Part model, mm, in its own coordinate system. Face numbers are marked on the shaded views. A direction names the side the tool comes from. Give positions to 0.01 mm unless a question says otherwise; leave off trailing zeros. Write each loop counter-clockwise with the first axis right and the second up, starting at its lowest first coordinate (ties: lowest second). Pieces come first, ordered by that corner, then holes. Notation, with made-up numbers: M -35,42 L 19,42 A33 cw 19,76 Z; hole C -7.75,-10 d3. An arc over 180 degrees is marked long. Use CSV: the item, a comma, the result in double quotes. Start each with the question number.
Item 1: Cut at A-A (x = -23). List the corners of the cut face in (y, z).
Item 2: Drill centre lines: line 1 (Z direction, x = -1, y = 37.5); line 2 (X direction, y = 141, z = 12); line 3 (Y direction, x = -45.5, z = 38). Where is each one in solid material? Low to high. Write a range as [from, to].
Item 3: Which spindle directions (+Z, -Z, +X, -X, +Y, -Y) get a long thin tool onto all of the face, cutting with end or side? Do the marked faces 1, 2, 3 and 4. Say none if no direction does.
Item 4: Cut at B-B (y = 90). List the corners of the cut face in (x, z), then the cut area to 3 significant figures.
Item 5: Cut at C-C (z = 99.5). List the corners of the cut face in (x, y), then the cut area to 3 significant figures.
Item 6: Pin check, flat tips, straight feed: pin 1 (5 mm diameter, centred on x = -51.49, z = 117.4, fed in from -Y); pin 2 (12.5 mm diameter, centred on y = 143.5, z = 36, fed in from +X); pin 3 (5 mm diameter, centred on x = 10.5, y = 35, fed in from +Z). Stop position of each tip, or through.
from build123d import *

# Parameters (mm, degrees)
SKETCH_1_W          = 120
SKETCH_1_H          = 20
EXTRUDE_1_DEPTH     = 150
SKETCH_2_W          = 90
SKETCH_2_H          = 25
EXTRUDE_2_DEPTH     = 130
SKETCH_3_R          = 2
CUT_EXTRUDE_1_DEPTH = 130
SKETCH_5_R          = 5
CUT_EXTRUDE_2_DEPTH = 17


with BuildPart() as part:
    # 草图1 → 凸台-拉伸1 (new body)
    with BuildSketch(Plane(origin=(0, 0, 0), x_dir=(1, 0, 0), z_dir=(0, 1, 0))):
        with Locations((-12.536231884, 9.565217391)):
            Rectangle(SKETCH_1_W, SKETCH_1_H)
    extrude(amount=EXTRUDE_1_DEPTH)

    # 草图2 → 凸台-拉伸2 (add)
    with BuildSketch(Plane.XY.offset(0.434782609)):
        with Locations((-13.26152797, 137.5)):
            Rectangle(SKETCH_2_W, SKETCH_2_H)
    extrude(amount=EXTRUDE_2_DEPTH)

    # 草图3 → 切除-拉伸1 (cut)
    with BuildSketch(Plane(origin=(0, 150, 0), x_dir=(1, 0, 0), z_dir=(0, 1, 0))):
        with Locations(Location((-51.492397045, -42.39796667, 0), (0, 0, 270))):
            Circle(SKETCH_3_R)
        with Locations(Location((23.507602913, -42.400462624, 0), (0, 0, 270))):
            Circle(SKETCH_3_R)
        with Locations(Location((-51.492397045, -117.400462624, 0), (0, 0, 270))):
            Circle(SKETCH_3_R)
        with Locations(Location((23.507602955, -117.400462624, 0), (0, 0, 270))):
            Circle(SKETCH_3_R)
    extrude(amount=-CUT_EXTRUDE_1_DEPTH, mode=Mode.SUBTRACT)

    # 草图5 → 切除-拉伸2 (cut)
    with BuildSketch(Plane.XZ.offset(-125)):
        with Locations((-51.492397045, 117.400462624)):
            Circle(SKETCH_5_R)
        with Locations((23.507602955, 117.400462624)):
            Circle(SKETCH_5_R)
        with Locations((23.507602913, 42.400462624)):
            Circle(SKETCH_5_R)
        with Locations((-51.492397045, 42.39796667)):
            Circle(SKETCH_5_R)
    extrude(amount=-CUT_EXTRUDE_2_DEPTH, mode=Mode.SUBTRACT)


solid = part.part
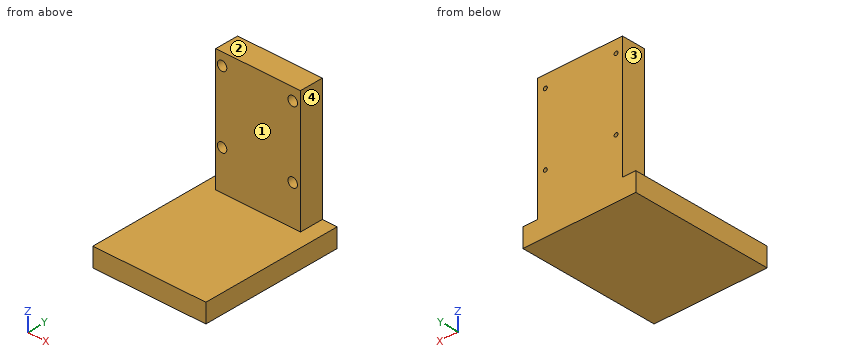
Worked answers:
1,outline,"M 0,-19.57 L 150,-19.57 L 150,130.43 L 125,130.43 L 125,0.43 L 0,0.43 Z"
2,line 1,"z = [-19.57, 0.43]"
2,line 2,"x = [-58.26, 31.74]"
2,line 3,"y = [125, 150]"
3,face 1,"+Z, +X, -X, -Y"
3,face 2,"+Z, +X, -X, +Y, -Y"
3,face 3,"+Z, -X, +Y, -Y"
3,face 4,"+Z, +X, +Y, -Y"
4,outline,"M -72.54,-19.57 L 47.46,-19.57 L 47.46,0.43 L -72.54,0.43 Z"
4,area,"2,400 mm^2"
5,outline,"M -58.26,125 L 31.74,125 L 31.74,150 L -58.26,150 Z"
5,area,"2,250 mm^2"
6,pin 1,"stops at y = 142"
6,pin 2,"stops at x = 31.74"
6,pin 3,"stops at z = 0.43"
